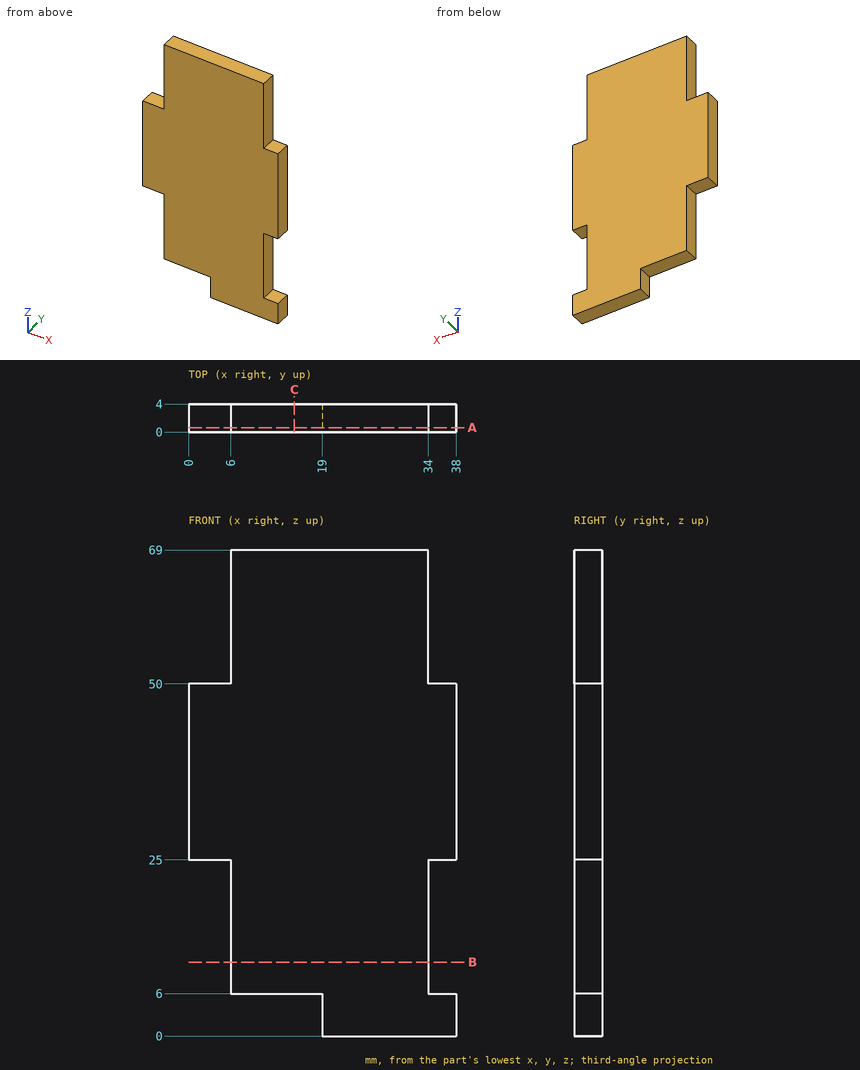
Verification items for this drawing (mm, ordinates from the low corner). Round coordinates to 2 decimals unless told otherwise and drop trailing zeros. Write each loop counter-clockwise with the first axis right and the second up, starting at its lowest first coordinate (ties: lowest second). Pieces come first, ordered by that corner, then holes. Notation, with made-up numbers: (18, 65) - (77, 65) arc R22 cw to (77, 91) - close; hole circle Ø5 at (59.25, -21). An arc over 180 degrees is marked (long way). Answer as a JSON object with one key per item and string values. Group by question number.
Q1. Go/stop test with flat-tipped pins: pin 1 Ø1 at (y, z) = (2.5, 56) entering from +X; pin 2 Ø2 at (y, z) = (2, 56) entering from -X; pin 3 Ø2 at (x, y) = (35.5, 1) entering from +Z. Record where each tip stops, or that it passes through.
Q2. Section check B-B, the plane z = 10.5. Enter the section's corners in (x, y), plus the area to 3 significant figures.
Q3. Section check C-C, the plane x = 15. Enter the section's corners in (y, z).
Q4. Section check A-A, the plane y = 0.65. Enter the section's corners in (x, z).
Q5. Thickness scan on line 1 (Z direction, x = 35, y = 0.2); line 2 (Z direction, x = 2.5, y = 2.2); line 3 (Z direction, x = 15, y = 2.35). Record the ranges inside material, lowest first.
Found:
{
 "1": {"pin 1": "stops at x = 34", "pin 2": "stops at x = 6", "pin 3": "stops at z = 50"},
 "2": {"outline": "(6, 0) - (34, 0) - (34, 4) - (6, 4) - close", "area": "112 mm^2"},
 "3": {"outline": "(0, 6) - (4, 6) - (4, 69) - (0, 69) - close"},
 "4": {"outline": "(0, 25) - (6, 25) - (6, 6) - (19, 6) - (19, 0) - (38, 0) - (38, 6) - (34, 6) - (34, 25) - (38, 25) - (38, 50) - (34, 50) - (34, 69) - (6, 69) - (6, 50) - (0, 50) - close"},
 "5": {"line 1": "z = 0 to 6, 25 to 50", "line 2": "z = 25 to 50", "line 3": "z = 6 to 69"}
}
